Input: part model. Units: mm. Frame: model coordinates. Face numbers are marked on the shaded views. A direction names the side the tool comes from. Coordinates: 2 decimals unless noted, no trailing zeros. Order: outer loops, then holes, each group sorted by start corner. A loop starts at its lowest first (then second) coordinate and runs counter-clockwise, first axis right, second up. Notation, with made-up numbers: (-20, 0) -> (8, 0) arc R34 ccw to (8, 33) -> close; hole circle Ø10 at (72.5, -5). An arc over 180 degrees is marked (long way). Write each question's results on one line, items separated by ' | '.
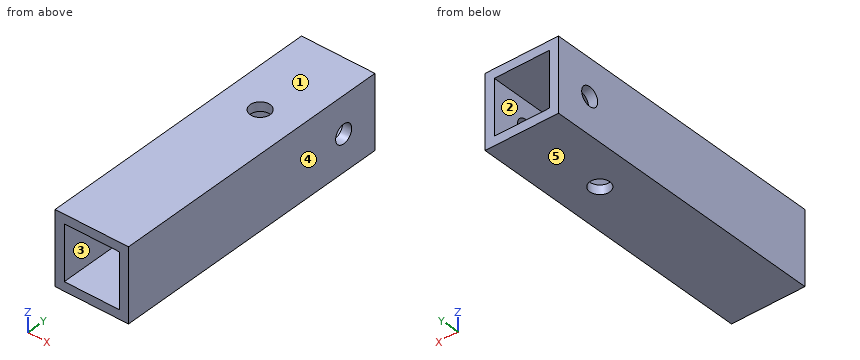
```python
from build123d import *

# Parameters (mm, degrees)
SKETCH1_W                = 25.4
SKETCH1_H                = 25.4
SKETCH1_W_2              = 19.05
SKETCH1_H_2              = 19.05
BOSS_EXTRUDE1_DEPTH      = 100.2538
F_0_257_DIAMETER_HOLE1_D = 6.5278
I_0_272_DIAMETER_HOLE1_D = 6.9088


with BuildPart() as part:
    # Sketch1 → Boss-Extrude1 (new body)
    with BuildSketch(Plane(origin=(0, 0, 0), x_dir=(1, 0, 0), z_dir=(0, 1, 0))):
        Rectangle(SKETCH1_W, SKETCH1_H)
        Rectangle(SKETCH1_W_2, SKETCH1_H_2, mode=Mode.SUBTRACT)
    extrude(amount=BOSS_EXTRUDE1_DEPTH)

    # F (0.257) Diameter Hole1 (through all)
    with Locations(Plane(origin=(12.7, 0, 0), x_dir=(0, 0, -1), z_dir=(1, 0, 0))):
        with Locations((0, 87.5538)):
            Hole(F_0_257_DIAMETER_HOLE1_D / 2)

    # I (0.272) Diameter Hole1 (through all)
    with Locations(Plane.XY.offset(12.7)):
        with Locations((0, 68.5038)):
            Hole(I_0_272_DIAMETER_HOLE1_D / 2)


solid = part.part
```
(1) Cut plane C-C, the plane z = 0. Return loops of the section in (x, y) (3 decimals).
Return value:
outline: (-12.7, 0) -> (-9.525, 0) -> (-9.525, 84.29) -> (-12.7, 84.29) -> close; (-12.7, 90.818) -> (-9.525, 90.818) -> (-9.525, 100.254) -> (-12.7, 100.254) -> close; (9.525, 0) -> (12.7, 0) -> (12.7, 84.29) -> (9.525, 84.29) -> close; (9.525, 90.818) -> (12.7, 90.818) -> (12.7, 100.254) -> (9.525, 100.254) -> close
(2) Cut plane A-A, the plane x = 0. Return loops of the section in (y, z) (3 decimals).
Return value:
outline: (0, -12.7) -> (65.049, -12.7) -> (65.049, -9.525) -> (0, -9.525) -> close; (0, 9.525) -> (65.049, 9.525) -> (65.049, 12.7) -> (0, 12.7) -> close; (71.958, -12.7) -> (100.254, -12.7) -> (100.254, -9.525) -> (71.958, -9.525) -> close; (71.958, 9.525) -> (100.254, 9.525) -> (100.254, 12.7) -> (71.958, 12.7) -> close
(3) Cut plane D-D, the plane x = 6. Return loops of the section in (y, z) (3 decimals), plus the area to 3 significant figures.
Return value:
outline: (0, -12.7) -> (100.254, -12.7) -> (100.254, -9.525) -> (0, -9.525) -> close; (0, 9.525) -> (100.254, 9.525) -> (100.254, 12.7) -> (0, 12.7) -> close | area: 637 mm2
(4) Reachability of the marked faces 1 and 2 from +Z, -Z, +X, -X, +Y, -Y: full face, straight path, thin tool, end or side. Return the list, or none.
Return value:
face 1: +Z, +X, -X, +Y, -Y | face 2: +Y, -Y
(5) Cut plane B-B, the plane y = 19. Return loops of the section in (x, z) (3 decimals).
Return value:
outline: (-12.7, -12.7) -> (12.7, -12.7) -> (12.7, 12.7) -> (-12.7, 12.7) -> close; hole (-9.525, -9.525) -> (9.525, -9.525) -> (9.525, 9.525) -> (-9.525, 9.525) -> close
(6) Line query: line 1 along Z through (x, y) = (-3, 62) (3 decimals); line 2 along Y through (x, z) = (11.8, 0). Output: solid intervals per line, ascending. Write a range as from..to.
Return value:
line 1: -12.7..-9.525, 9.525..12.7 | line 2: 0..84.29, 90.82..100.25
(7) Mould query, pull axis X, two halves, no side actions, for the marked faces 3, 4 and 5. Classes: +X half, -X half, draft (parallel to the pull), parting line (faces both ways), or undercut.
Return value:
face 3: undercut | face 4: +X half | face 5: draft
